```python
from build123d import *

# Parameters (mm, degrees)
SZKIC1_R                    = 5
DODANIE_WYCI_GNI_CIE1_DEPTH = 25
OTW_R_3_2_3_2_1_D           = 3.2
OTW_R_3_2_3_2_1_DEPTH       = 5
OTW_R_3_2_3_2_1_TIP         = 0.96137699


with BuildPart() as part:
    # Szkic1 → Dodanie-wyciągnięcie1 (new body)
    with BuildSketch(Plane.XY):
        with BuildLine():
            Line((-7, -5), (-7, 0))
            Line((-7, 0), (-12.5, 0))
            Line((-12.5, 0), (-12.5, 5))
            Line((-12.5, 5), (12.5, 5))
            Line((12.5, 5), (12.5, 0))
            Line((12.5, 0), (7, 0))
            Line((7, 0), (7, -5))
            ThreePointArc((7, -5), (0, -12), (-7, -5))
        make_face()
        with Locations((0, -5)):
            Circle(SZKIC1_R, mode=Mode.SUBTRACT)
    extrude(amount=DODANIE_WYCI_GNI_CIE1_DEPTH)

    # Otwór Ø3.2 (3.2)1
    with Locations(Plane.XZ):
        with Locations((9.75, 19.5), (-9.75, 19.5), (-9.75, 5.5), (9.75, 5.5)):
            Hole(OTW_R_3_2_3_2_1_D / 2, depth=OTW_R_3_2_3_2_1_DEPTH)
            with Locations((0, 0, -(OTW_R_3_2_3_2_1_DEPTH + OTW_R_3_2_3_2_1_TIP / 2))):  # 118° drill point
                Cone(0, OTW_R_3_2_3_2_1_D / 2, OTW_R_3_2_3_2_1_TIP, mode=Mode.SUBTRACT)


solid = part.part
```
Design review of the part built by this model. Coordinates are the model's own, in mm. A direction names the side the tool comes from. Round coordinates to 2 decimals unless told otherwise and drop trailing zeros. Write each loop counter-clockwise with the first axis right and the second up, starting at its lowest first coordinate (ties: lowest second). Pieces come first, ordered by that corner, then holes. Notation, with made-up numbers: (-12.75, 34) -> (5.25, 34) arc R13 ccw to (5.25, 55) -> close; hole circle Ø6 at (33, 85). An arc over 180 degrees is marked (long way). Answer in a Markdown table with one row per item.
Q1. For faces 1 (the face through (10, 0, 12)), 2 (the face through (-8.15, 2.54, 5.57)), 3 (the face through (-10, 0, 12)), list the 3-axis set-ups (+Z, -Z, +X, -X, +Y, -Y) from which the entire face can be reached by the end or side of a thin tool; tool diameter is ignored.
The answers:
| item | result |
|---|---|
| face 1 | +Z, -Z, +X, -Y |
| face 2 | +Y, -Y |
| face 3 | +Z, -Z, -X, -Y |
Q2. Take a section at A-A, the plane z = 19.5. State the section outline as (x, y) points, then the cut area to 3 significant figures.
The answers:
| item | result |
|---|---|
| outline | (-12.5, 0) -> (-11.35, 0) -> (-11.35, 5) -> (-12.5, 5) -> close; (-8.15, 0) -> (-7, 0) -> (-7, -5) arc R7 ccw to (7, -5) -> (7, 0) -> (8.15, 0) -> (8.15, 5) -> (-8.15, 5) -> close; (11.35, 0) -> (12.5, 0) -> (12.5, 5) -> (11.35, 5) -> close; hole circle Ø10 at (0, -5) |
| area | 161 mm² |
Q3. To check wall thickness, follow L1, parallel to Z at x = -9.75, y = 2.45; L2, parallel to Y at x = -7.5, z = 11; L3, parallel to X at y = -9, z = 18.5. State the ranges of each line that lie inside material, in increasing order. Write a range as [from, to].
The answers:
| item | result |
|---|---|
| L1 | [0, 3.9], [7.1, 17.9], [21.1, 25] |
| L2 | [0, 5] |
| L3 | [-5.74, -3], [3, 5.74] |
Q4. Take a section at D-D, the plane x = 9.75. State the section outline as (y, z) points, then the cut area to 3 significant figures.
The answers:
| item | result |
|---|---|
| outline | (0, 0) -> (5, 0) -> (5, 3.9) -> (0, 3.9) -> close; (0, 7.1) -> (5, 7.1) -> (5, 17.9) -> (0, 17.9) -> close; (0, 21.1) -> (5, 21.1) -> (5, 25) -> (0, 25) -> close |
| area | 93.0 mm² |
Q5. Clearance check with flat-ended pins moving along their axes: pin 1 Ø2.5 at (x, z) = (-9.75, 5.5) entering from -Y; pin 2 Ø1.6 at (x, z) = (-9.5, 16.5) entering from -Y; pin 3 Ø1 at (x, z) = (-6, 17) entering from -Y. State where each tip first meets the part, or that it passes through.
The answers:
| item | result |
|---|---|
| pin 1 | through |
| pin 2 | y = 0 |
| pin 3 | y = -9.33 |
Q6. Draft analysis for pull direction X (two halves, no side actions). For faces 4 (the face through (0.2, 0.4, 25)), 5 (the face through (12.5, 3, 12)), 6 (the face through (9.958, 2.535, 21.086)), 7 (the face through (-7, -3, 12)), state which applies: +X half, -X half, draft (parallel to the pull), parting line (faces both ways), or undercut.
The answers:
| item | result |
|---|---|
| face 4 | draft |
| face 5 | +X half |
| face 6 | undercut |
| face 7 | -X half |
Q7. Take a section at C-C, the plane y = 0.75. State the section outline as (x, z) points, then the cut area to 3 significant figures.
The answers:
| item | result |
|---|---|
| outline | (-12.5, 0) -> (12.5, 0) -> (12.5, 25) -> (-12.5, 25) -> close; hole circle Ø3.2 at (-9.75, 5.5); hole circle Ø3.2 at (-9.75, 19.5); hole circle Ø3.2 at (9.75, 5.5); hole circle Ø3.2 at (9.75, 19.5) |
| area | 593 mm² |
Q8. Take a section at B-B, the plane x = 0. State the section outline as (y, z) points, then the cut area to 3 significant figures.
The answers:
| item | result |
|---|---|
| outline | (-12, 0) -> (-10, 0) -> (-10, 25) -> (-12, 25) -> close; (0, 0) -> (5, 0) -> (5, 25) -> (0, 25) -> close |
| area | 175 mm² |
